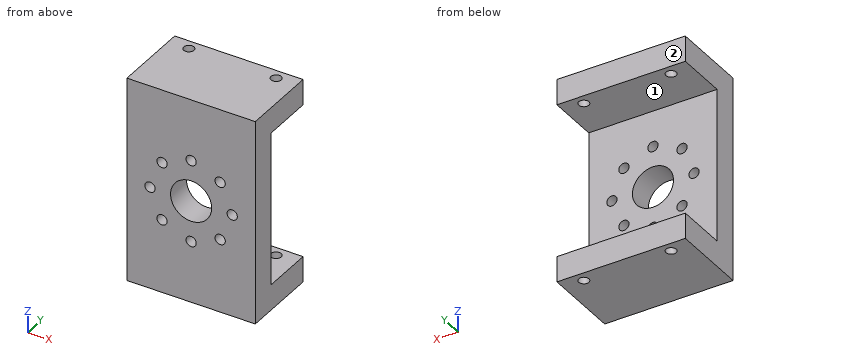
```python
from build123d import *

# Parameters (mm, degrees)
SKETCH1_W           = 25
SKETCH1_H           = 40
BOSS_EXTRUDE1_DEPTH = 5
SKETCH5_W           = 25
SKETCH5_H           = 5
BOSS_EXTRUDE2_DEPTH = 10
SKETCH6_R           = 1
CUT_EXTRUDE3_DEPTH  = 45.511234537
SKETCH7_R           = 4
SKETCH7_R_2         = 1
CUT_EXTRUDE4_DEPTH  = 10


with BuildPart() as part:
    # Sketch1 → Boss-Extrude1 (new body)
    with BuildSketch(Plane(origin=(0, 0, 0), x_dir=(1, 0, 0), z_dir=(0, 1, 0))):
        Rectangle(SKETCH1_W, SKETCH1_H)
    extrude(amount=BOSS_EXTRUDE1_DEPTH)

    # Sketch5 → Boss-Extrude2 (add)
    with BuildSketch(Plane(origin=(0, 5, 0), x_dir=(1, 0, 0), z_dir=(0, 1, 0))):
        with Locations((0, 17.5)):
            Rectangle(SKETCH5_W, SKETCH5_H)
        with Locations((0, -17.5)):
            Rectangle(SKETCH5_W, SKETCH5_H)
    extrude(amount=BOSS_EXTRUDE2_DEPTH)

    # Sketch6 → Cut-Extrude3 (cut, through all)
    with BuildSketch(Plane.XY.offset(20)):
        with Locations((-8.5, 13)):
            Circle(SKETCH6_R)
        with Locations((8.5, 13)):
            Circle(SKETCH6_R)
    extrude(amount=-CUT_EXTRUDE3_DEPTH, mode=Mode.SUBTRACT)

    # Sketch7 → Cut-Extrude4 (cut)
    with BuildSketch(Plane.XZ):
        with Locations(Location((0, 0, 0), (0, 0, 270))):
            Circle(SKETCH7_R)
        with Locations(Location((0, 8, 0), (0, 0, 270))):
            Circle(SKETCH7_R_2)
        with Locations(Location((5.656854249, 5.656854249, 0), (0, 0, 270))):
            Circle(SKETCH7_R_2)
        with Locations(Location((8, 0, 0), (0, 0, 270))):
            Circle(SKETCH7_R_2)
        with Locations(Location((5.656854249, -5.656854249, 0), (0, 0, 270))):
            Circle(SKETCH7_R_2)
        with Locations(Location((0, -8, 0), (0, 0, 270))):
            Circle(SKETCH7_R_2)
        with Locations(Location((-5.656854249, -5.656854249, 0), (0, 0, 270))):
            Circle(SKETCH7_R_2)
        with Locations(Location((-8, 0, 0), (0, 0, 270))):
            Circle(SKETCH7_R_2)
        with Locations(Location((-5.656854249, 5.656854249, 0), (0, 0, 270))):
            Circle(SKETCH7_R_2)
    extrude(amount=-CUT_EXTRUDE4_DEPTH, mode=Mode.SUBTRACT)


solid = part.part
```
Input: part model. Units: mm. Frame: model coordinates. Face numbers are marked on the shaded views. A direction names the side the tool comes from. Give positions to 0.01 mm unless a question says otherwise; leave off trailing zeros. Order: outer loops, then holes, each group sorted by start corner. A loop starts at its lowest first (then second) coordinate and runs counter-clockwise, first axis right, second up. Notation, with made-up numbers: (78, 15.5) - (98, 15.5) arc R28 ccw to (98, 41.5) - close; hole circle Ø9 at (-19, 72.25). An arc over 180 degrees is marked (long way). Put each result on its own line as item: value.
Item 1: Ray query, L1, parallel to X at y = 1.5, z = 0; L2, parallel to Z at x = 3.25, y = 12.75; L3, parallel to Y at x = 8.5, z = 17.85. Return the intervals inside material, ascending. Write a range as from..to.
Found:
L1: x = -12.5..-9, -7..-4, 4..7, 9..12.5
L2: z = -20..-15, 15..20
L3: y = 0..12, 14..15
Item 2: Contact query for a flat-ended pin moving along its axis: pin 1 (3 mm diameter, centred on x = 5.66, z = 5.66, fed in from +Y). Output: stop coordinate, or through.
Found:
pin 1: stops at y = 5
Item 3: Section query D-D, the plane z = 0. Return loops of the section in (x, y), then the cut area to 3 significant figures.
Found:
outline: (-12.5, 0) - (-9, 0) - (-9, 5) - (-12.5, 5) - close; (-7, 0) - (-4, 0) - (-4, 5) - (-7, 5) - close; (4, 0) - (7, 0) - (7, 5) - (4, 5) - close; (9, 0) - (12.5, 0) - (12.5, 5) - (9, 5) - close
area: 65.0 mm^2
Item 4: Section query A-A, the plane y = 8.5. Return loops of the section in (x, z).
Found:
outline: (-12.5, -20) - (12.5, -20) - (12.5, -15) - (-12.5, -15) - close; (-12.5, 15) - (12.5, 15) - (12.5, 20) - (-12.5, 20) - close
Item 5: Section query B-B, the plane z = -8. Return loops of the section in (x, y), then the cut area to 3 significant figures.
Found:
outline: (-12.5, 0) - (-1, 0) - (-1, 5) - (-12.5, 5) - close; (1, 0) - (12.5, 0) - (12.5, 5) - (1, 5) - close
area: 115 mm^2
Item 6: Section query C-C, the plane y = 13. Return loops of the section in (x, z).
Found:
outline: (-12.5, -20) - (-9.5, -20) - (-9.5, -15) - (-12.5, -15) - close; (-12.5, 15) - (-9.5, 15) - (-9.5, 20) - (-12.5, 20) - close; (-7.5, -20) - (7.5, -20) - (7.5, -15) - (-7.5, -15) - close; (-7.5, 15) - (7.5, 15) - (7.5, 20) - (-7.5, 20) - close; (9.5, -20) - (12.5, -20) - (12.5, -15) - (9.5, -15) - close; (9.5, 15) - (12.5, 15) - (12.5, 20) - (9.5, 20) - close
Item 7: Access query for the marked faces 1 and 2. Directions: +Z, -Z, +X, -X, +Y, -Y. A direction counts if a zero-diameter tool reaches every point of the face in a straight line with its end or side. Return the directions, or none.
Found:
face 1: +X, -X, +Y
face 2: +Z, -Z, +X, -X, +Y
